```python
from build123d import *

# Parameters (mm, degrees)
BOSS_EXTRU_1_DEPTH      = 8
ESQUISSE2_R             = 2
ENL_V_MAT_EXTRU_1_DEPTH = 10
ESQUISSE3_R             = 2
ENL_V_MAT_EXTRU_2_DEPTH = 39.745967532
CHANFREIN1_SIZE         = 2.5
ESQUISSE4_R             = 8
ENL_V_MAT_EXTRU_3_DEPTH = 5
ESQUISSE5_R             = 3
ENL_V_MAT_EXTRU_4_DEPTH = 39.23937761
ESQUISSE6_W             = 50
ESQUISSE6_H             = 8
ENL_V_MAT_EXTRU_5_DEPTH = 4
CONG_1_R                = 3.5


with BuildPart() as part:
    # Esquisse1 → Boss.-Extru.1 (new body)
    with BuildSketch(Plane.XY):
        Polygon((-25, -23.5), (-20, -23.5), (-20, -28.5), (20, -28.5), (20, -23.5), (25, -23.5), (25, 28.5), (-25, 28.5), align=None)
    extrude(amount=BOSS_EXTRU_1_DEPTH)

    # Esquisse2 → Enlèv. mat.-Extru.1 (cut)
    with BuildSketch(Plane.XZ.offset(28.5)):
        with Locations(Location((-15, 4, 0), (0, 0, 270))):
            Circle(ESQUISSE2_R)
        with Locations(Location((15, 4, 0), (0, 0, 270))):
            Circle(ESQUISSE2_R)
    extrude(amount=-ENL_V_MAT_EXTRU_1_DEPTH, mode=Mode.SUBTRACT)

    # Esquisse3 → Enlèv. mat.-Extru.2 (cut, through all)
    with BuildSketch(Plane.XY.offset(8)):
        with Locations((-20, 24.5)):
            Circle(ESQUISSE3_R)
        with Locations((20, 24.5)):
            Circle(ESQUISSE3_R)
        with Locations((0, 24.5)):
            Circle(ESQUISSE3_R)
    extrude(amount=-ENL_V_MAT_EXTRU_2_DEPTH, mode=Mode.SUBTRACT)

    # Chanfrein1
    # the kernel refuses this chamfer: 2.5 mm, written as the material it takes off along each edge
    with BuildSketch(Plane(origin=(-20, 24.5, 0), x_dir=(1, 0, 0), z_dir=(0, -1, 0))) as chanfrein1_piece_1:
        Polygon((2 + CHANFREIN1_SIZE, 0), (2, CHANFREIN1_SIZE), (2, 0), align=None)
    revolve(axis=Axis((-20, 24.5, 0), (0, 0, 1)), mode=Mode.SUBTRACT)
    with BuildSketch(Plane(origin=(20, 24.5, 0), x_dir=(1, 0, 0), z_dir=(0, -1, 0))) as chanfrein1_piece_2:
        Polygon((2 + CHANFREIN1_SIZE, 0), (2, CHANFREIN1_SIZE), (2, 0), align=None)
    revolve(axis=Axis((20, 24.5, 0), (0, 0, 1)), mode=Mode.SUBTRACT)
    with BuildSketch(Plane(origin=(0, 24.5, 0), x_dir=(1, 0, 0), z_dir=(0, -1, 0))) as chanfrein1_piece_3:
        Polygon((2 + CHANFREIN1_SIZE, 0), (2, CHANFREIN1_SIZE), (2, 0), align=None)
    revolve(axis=Axis((0, 24.5, 0), (0, 0, 1)), mode=Mode.SUBTRACT)

    # Esquisse4 → Enlèv. mat.-Extru.3 (cut)
    with BuildSketch(Plane.XY.offset(8)):
        with Locations((0, -12.5)):
            Circle(ESQUISSE4_R)
    extrude(amount=-ENL_V_MAT_EXTRU_3_DEPTH, mode=Mode.SUBTRACT)

    # Esquisse5 → Enlèv. mat.-Extru.4 (cut, through all)
    with BuildSketch(Plane.XY.offset(3)):
        with Locations((0, -12.5)):
            Circle(ESQUISSE5_R)
    extrude(amount=-ENL_V_MAT_EXTRU_4_DEPTH, mode=Mode.SUBTRACT)

    # Esquisse6 → Enlèv. mat.-Extru.5 (cut)
    with BuildSketch(Plane.XY.offset(8)):
        with Locations((0, 24.5)):
            Rectangle(ESQUISSE6_W, ESQUISSE6_H)
    extrude(amount=-ENL_V_MAT_EXTRU_5_DEPTH, mode=Mode.SUBTRACT)

    # Congé1
    cong_1_edges = [part.edges().sort_by_distance(p)[0] for p in [
        (20, -23.5, 4),
        (-20, -23.5, 4),
    ]]
    fillet(cong_1_edges, radius=CONG_1_R)


solid = part.part
```
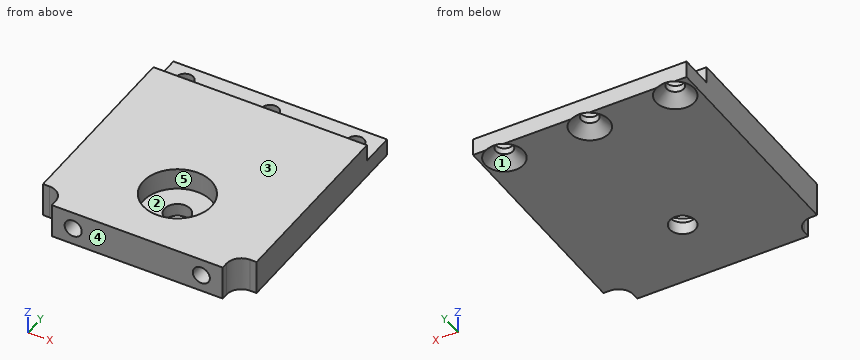
CAD build for the part. Positions are in the model's coordinates, mm. Face numbers are marked on the shaded views. A direction names the side the tool comes from. Coordinates: 2 decimals unless noted, no trailing zeros. Loops run counter-clockwise (first coordinate to the right, second up) from the corner with the lowest first, then second, coordinate; pieces in that order, holes last. Notation, with made-up numbers: (26, -18.75) - (32, -18.75) arc R27 cw to (32, 3.25) - close; hole circle Ø11 at (34, 24). An arc over 180 degrees is marked (long way). Return JSON: item names as keys, results as strings.
1. Mould opens along Y. For the marked faces 3, 4 and 5 say: released by +Y, released by -Y, zero draft, split by the parting line, or undercut.
Result:
{"face 3": "zero draft", "face 4": "released by -Y", "face 5": "undercut"}
2. Drop flat-ended pins along their axis: pin 1 (13 mm diameter, centred on x = 0, y = -12.5, fed in from +Z); pin 2 (2 mm diameter, centred on y = 21, z = 5, fed in from -X); pin 3 (1.2 mm diameter, centred on x = 14, z = 3.5, fed in from -Y); pin 4 (0.8 mm diameter, centred on x = 24.5, z = 5.5, fed in from -Y). Give the stop position or say it passes through.
Result:
{"pin 1": "stops at z = 3", "pin 2": "stops at x = -25", "pin 3": "stops at y = -18.5", "pin 4": "stops at y = -23.5"}
3. Band-saw the part on B-B (x = 0). Give the cut face in (y, z), and give its area (3 significant figures).
Result:
{"outline": "(-28.5, 0) - (-15.5, 0) - (-15.5, 3) - (-20.5, 3) - (-20.5, 8) - (-28.5, 8) - close; (-9.5, 0) - (20, 0) - (22.5, 2.5) - (22.5, 4) - (20.5, 4) - (20.5, 8) - (-4.5, 8) - (-4.5, 3) - (-9.5, 3) - close; (26.5, 2.5) - (28.5, 0.5) - (28.5, 4) - (26.5, 4) - close", "area": "304 mm2"}
4. Band-saw the part on D-D (y = -12.5). Give the cut face in (x, z).
Result:
{"outline": "(-25, 0) - (-3, 0) - (-3, 3) - (-8, 3) - (-8, 8) - (-25, 8) - close; (3, 0) - (25, 0) - (25, 8) - (8, 8) - (8, 3) - (3, 3) - close"}
5. Probe L1, parallel to X at y = -22, z = 4; L2, parallel to Y at x = 0, z = 4.55; L3, parallel to X at y = -25.75, z = 4. List the from-to ranges inside material, lowest first. Write a range as from..to.
Result:
{"L1": "x = -25..-17, -13..13, 17..25", "L2": "y = -28.5..-20.5, -4.5..20.5", "L3": "x = -20.23..-17, -13..13, 17..20.23"}
6. Band-saw the part on C-C (y = 24.5). Give the cut face in (x, z).
Result:
{"outline": "(-25, 0) - (-24.5, 0) - (-22, 2.5) - (-22, 4) - (-25, 4) - close; (-18, 2.5) - (-15.5, 0) - (-4.5, 0) - (-2, 2.5) - (-2, 4) - (-18, 4) - close; (2, 2.5) - (4.5, 0) - (15.5, 0) - (18, 2.5) - (18, 4) - (2, 4) - close; (22, 2.5) - (24.5, 0) - (25, 0) - (25, 4) - (22, 4) - close"}
7. 3-axis set-ups, long thin cutter, end or side, ignore diameter. For the marked faces 1 and 2: which of +Z, -Z, +X, -X, +Y, -Y reach the whole face in a straight line?
Result:
{"face 1": "-Z", "face 2": "+Z"}
8. Band-saw the part on A-A (z = 1.25). Give the cut face in (x, y).
Result:
{"outline": "(-25, -23.5) - (-23.5, -23.5) arc R3.5 cw to (-20, -27) - (-20, -28.5) - (20, -28.5) - (20, -27) arc R3.5 cw to (23.5, -23.5) - (25, -23.5) - (25, 28.5) - (-25, 28.5) - close; hole circle Ø6.5 at (-20, 24.5); hole circle Ø6.5 at (0, 24.5); hole circle Ø6 at (0, -12.5); hole circle Ø6.5 at (20, 24.5)"}
